```python
from build123d import *

# Parameters (mm, degrees)
ESQUISSE1_W             = 32
ESQUISSE1_H             = 66
BOSS_EXTRU_1_DEPTH      = 5
ENL_V_MAT_EXTRU_1_DEPTH = 1


with BuildPart() as part:
    # Esquisse1 → Boss.-Extru.1 (new body)
    with BuildSketch(Plane.XY):
        Rectangle(ESQUISSE1_W, ESQUISSE1_H)
    extrude(amount=BOSS_EXTRU_1_DEPTH)

    # Esquisse2 → Enlèv. mat.-Extru.1 (cut)
    with BuildSketch(Plane.XY.offset(5)):
        with BuildLine():
            Line((-10.020527486, -11.48471415), (-12.020211327, -11.449153833))
            ThreePointArc((-12.020211327, -11.449153833), (-0.228779166, -23.452136955), (11.562652994, -11.449153833))
            Line((11.562652994, -11.449153833), (9.562969153, -11.48471415))
            ThreePointArc((9.562969153, -11.48471415), (-0.228779166, -21.452136955), (-10.020527486, -11.48471415))
        make_face()
        Polygon((11.562652994, -7.092154157), (-12.020211327, -0.686337499), (11.562652994, 9.837504153), (12.377681975, 8.011106671), (-6.082483824, -0.226733274), (12.086916587, -5.162089991), align=None)
        Polygon((11.562652994, 12.765877482), (-12.020211327, 19.263205806), (5.170409159, 23.015184134), (-12.020211327, 27.751381734), (-11.488983181, 29.679540611), (13.517651309, 22.78994856), (-3.672969177, 19.037970232), (12.09388114, 14.694036359), align=None)
    extrude(amount=-ENL_V_MAT_EXTRU_1_DEPTH, mode=Mode.SUBTRACT)


solid = part.part
```
The listing builds one solid part. Answer for the finished solid, in the listing's coordinates (mm). A direction names the side the tool comes from. Round coordinates to 2 decimals unless told otherwise and drop trailing zeros. Order: outer loops, then holes, each group sorted by start corner. A loop starts at its lowest first (then second) coordinate and runs counter-clockwise, first axis right, second up. Notation, with made-up numbers: (63, -6.75) -> (82, -6.75) arc R5 ccw to (82, -0.75) -> close; hole circle Ø2 at (-31.75, 71). An arc over 180 degrees is marked (long way). Answer as CSV lines item,"result". Start each with the question number.
(1) The part is cut by section D-D (y = -15). Determine the outline of the cut face in (x, z), then the cut area to 3 significant figures.
(2) The part is cut by section A-A (x = 8). Determine the outline of the cut face in (y, z).
(3) Find the intervals of material crossed by probe 1 along Z at (x, y) = (-5.5, -20.5); probe 2 along Y at (x, z) = (7.5, 4.45); probe 3 along Y at (x, z) = (10.5, 4.35), in increasing order. Write a range as from..to.
(4) A flat-ended cylindrical pin translates along its axis: pin 1 Ø13.5 at (x, y) = (3.5, 22) entering from +Z. Find the tip coordinate at first contact, or state that the pin passes through.
(5) A tool of negligible diameter and unlimited length cuts with its end or side. For faces 1 (the face through (4.1, 16.896, 4.507)), 2 (the face through (-16, 0, 2)), from which of +Z, -Z, +X, -X, +Y, -Y can it reach the whole face along a straight path? Write none if from no direction.
(6) For a pull along Y with two mould halves and no side action, classify faces 3 (the face through (16, 0, 2)), 4 (the face through (-0.01, -21.45, 4.51)), 5 (the face through (-0.06, 15.97, 4.51)), 6 (the face through (0, -33, 2)) as +Y half, -Y half, draft (parallel to the pull), parting line (faces both ways), or undercut.
(7) The part is cut by section B-B (y = 22). Determine the outline of the cut face in (x, z), then the cut area to 3 significant figures.
(8) The part is cut by section C-C (x = -8.5). Determine the outline of the cut face in (y, z).
Evaluation:
1,outline,"(-16, 0) -> (16, 0) -> (16, 5) -> (11.08, 5) -> (11.08, 4) -> (8.98, 4) -> (8.98, 5) -> (-9.43, 5) -> (-9.43, 4) -> (-11.54, 4) -> (-11.54, 5) -> (-16, 5) -> close"
1,area,"156 mm²"
2,outline,"(-33, 0) -> (33, 0) -> (33, 5) -> (24.31, 5) -> (24.31, 4) -> (21.59, 4) -> (21.59, 5) -> (15.82, 5) -> (15.82, 4) -> (13.75, 4) -> (13.75, 5) -> (8.25, 5) -> (8.25, 4) -> (6.06, 4) -> (6.06, 5) -> (-4.05, 5) -> (-4.05, 4) -> (-6.12, 4) -> (-6.12, 5) -> (-16.97, 5) -> (-16.97, 4) -> (-20.11, 4) -> (-20.11, 5) -> (-33, 5) -> close"
3,probe 1,"0..4"
3,probe 2,"-33..-20.57, -17.67..-5.99, -3.92..5.83, 8.02..13.89, 15.96..21.48, 24.45..33"
3,probe 3,"-33..-16.56, -11.47..-6.8, -4.73..7.17, 9.36..13.06, 15.13..22.13, 23.62..33"
4,pin 1,"z = 5"
5,face 1,"+Z"
5,face 2,"+Z, -Z, -X, +Y, -Y"
6,face 3,"draft"
6,face 4,"undercut"
6,face 5,"undercut"
6,face 6,"-Y half"
7,outline,"(-16, 0) -> (16, 0) -> (16, 5) -> (9.9, 5) -> (9.9, 4) -> (0.52, 4) -> (0.52, 5) -> (-16, 5) -> close"
7,area,"151 mm²"
8,outline,"(-33, 0) -> (33, 0) -> (33, 5) -> (28.86, 5) -> (28.86, 4) -> (26.78, 4) -> (26.78, 5) -> (20.03, 5) -> (20.03, 4) -> (18.29, 4) -> (18.29, 5) -> (0.88, 5) -> (0.88, 4) -> (-1.64, 4) -> (-1.64, 5) -> (-16.9, 5) -> (-16.9, 4) -> (-20.07, 4) -> (-20.07, 5) -> (-33, 5) -> close"
